from build123d import *

# Parameters (mm, degrees)
F0_R           = 13.97
F0_R_2         = 3.9751
F1_DEPTH       = 15.367
F3_D           = 2.9464
F3_CBORE_D     = 4.572
F3_CBORE_DEPTH = 6.35
F4_R           = 6.4135
F4_R_2         = 3.9751
F5_DEPTH       = 2.54
F6_R           = 1.27
F8_R           = 13.97
F8_R_2         = 12.7
F9_DEPTH       = 10.541


with BuildPart() as f1:
    # F0 (on Front) → F1 (new body)
    with BuildSketch(Plane.XZ):
        Circle(F0_R)
        Circle(F0_R_2, mode=Mode.SUBTRACT)
    extrude(amount=F1_DEPTH)

    # F3 (through all)
    with Locations(Plane.XZ.offset(15.367)):
        with Locations((0, 8.89), (-7.6989658396, -4.445), (7.6989658396, -4.445)):
            CounterBoreHole(F3_D / 2, F3_CBORE_D / 2, F3_CBORE_DEPTH)

    # F4 (on face) → F5 (cut)
    with BuildSketch(Plane(origin=(0, 0, 0), x_dir=(-1, 0, 0), z_dir=(0, 1, 0))):
        Circle(F4_R)
        Circle(F4_R_2, mode=Mode.SUBTRACT)
    extrude(amount=-F5_DEPTH, mode=Mode.SUBTRACT)

    # F7: sweep along a path in F7_path
    with BuildLine(Plane(origin=(13.97, -15.367, 0), x_dir=(0, 0, -1), z_dir=(0, 1, 0))) as f7_path:
        CenterArc((0, 13.97), 13.97, 0, 360)
    # F6 (on Right) → F7 (sweep, cut)
    with BuildSketch(Plane.YZ):
        with Locations((-12.954, 13.97)):
            Circle(F6_R)
    sweep(path=f7_path.line, mode=Mode.SUBTRACT)

    # F8 (on face) → F9 (cut)
    with BuildSketch(Plane(origin=(0, 0, 0), x_dir=(-1, 0, 0), z_dir=(0, 1, 0))):
        Circle(F8_R)
        Circle(F8_R_2, mode=Mode.SUBTRACT)
    extrude(amount=-F9_DEPTH, mode=Mode.SUBTRACT)


solid = f1.part
Geometry check sheet. Reference: the model listing, model coordinates, mm. A direction names the side the tool comes from. Round coordinates to 2 decimals unless told otherwise and drop trailing zeros. Loops run counter-clockwise (first coordinate to the right, second up) from the corner with the lowest first, then second, coordinate; pieces in that order, holes last. Notation, with made-up numbers: (-16, -15) -> (7, -15) arc R14 ccw to (7, -3) -> close; hole circle Ø9 at (-22.5, 45). An arc over 180 degrees is marked (long way). Answer as a JSON object with one key per item and string values. Group by question number.
Item 1: Cross-section at C-C, the plane y = -11.25. Record the cut outline in (x, z) (3 decimals), plus the area to 3 significant figures.
Item 2: Cross-section at A-A, the plane z = 0. Record the cut outline in (x, y), plus the area to 3 significant figures.
Item 3: Cross-section at B-B, the plane x = 0. Record the cut outline in (y, z).
Item 4: Set-up check for faces 1 (the face through (-8.38, -4.45, -5.75)), 2 (the face through (-3, -2.54, 3)), 3 (the face through (-6, -9.017, -4)): record each of +Z, -Z, +X, -X, +Y, -Y from which the full face is reachable in a straight line by a thin tool's end or side.
Item 5: Cross-section at D-D, the plane y = -9.5. Record the cut outline in (x, z) (3 decimals), plus the area to 3 significant figures.
Item 6: Release check for a two-part mould opening along X. For faces 4 (the face through (13.325, -11.104, 4.196)), 5 (the face through (3, -15.367, -3)), 6 (the face through (-6.5, -12.2, -2.5)) record: pulls with the +X half, pulls with the -X half, needs draft (parallel to the pull), parting line crosses it, or undercut.
Item 7: Thickness scan on line 1 along Z through (x, y) = (0, -2); line 2 along Z through (x, y) = (0, -6.5); line 3 along X through (y, z) = (-2.5, -3.75). Record the ranges inside material, lowest first.
Item 8: Depth check by flat-ended pin: pin 1 Ø3.5 at (x, z) = (-7.7, -4.44) entering from -Y; pin 2 Ø12.5 at (x, z) = (0, 0) entering from +Y; pin 3 Ø5 at (x, y) = (-5.5, -4) entering from +Z. Enter the tip coordinate at first touch or a pass-through.
Determined:
{
 "1": {"outline": "circle Ø27.94 at (0, 0); hole circle Ø4.572 at (-7.699, -4.445); hole circle Ø7.95 at (0, 0); hole circle Ø4.572 at (0, 8.89); hole circle Ø4.572 at (7.699, -4.445)", "area": "514 mm²"},
 "2": {"outline": "(-13.97, -15.37) -> (-3.98, -15.37) -> (-3.98, -2.54) -> (-6.41, -2.54) -> (-6.41, 0) -> (-12.7, 0) -> (-12.7, -10.54) -> (-13.97, -10.54) -> (-13.97, -11.68) arc R1.27 cw to (-13.97, -14.22) -> close; (3.98, -15.37) -> (13.97, -15.37) -> (13.97, -14.22) arc R1.27 cw to (13.97, -11.68) -> (13.97, -10.54) -> (12.7, -10.54) -> (12.7, 0) -> (6.41, 0) -> (6.41, -2.54) -> (3.98, -2.54) -> close", "area": "263 mm²"},
 "3": {"outline": "(-15.37, -13.97) -> (-14.22, -13.97) arc R1.27 cw to (-11.68, -13.97) -> (-10.54, -13.97) -> (-10.54, -12.7) -> (0, -12.7) -> (0, -6.41) -> (-2.54, -6.41) -> (-2.54, -3.98) -> (-15.37, -3.98) -> close; (-15.37, 3.98) -> (-2.54, 3.98) -> (-2.54, 6.41) -> (0, 6.41) -> (0, 7.42) -> (-9.02, 7.42) -> (-9.02, 6.6) -> (-15.37, 6.6) -> close; (-15.37, 11.18) -> (-9.02, 11.18) -> (-9.02, 10.36) -> (0, 10.36) -> (0, 12.7) -> (-10.54, 12.7) -> (-10.54, 13.97) -> (-11.68, 13.97) arc R1.27 cw to (-14.22, 13.97) -> (-15.37, 13.97) -> close"},
 "4": {"face 1": "+Y, -Y", "face 2": "+Y", "face 3": "-Y"},
 "5": {"outline": "circle Ø25.4 at (0, 0); hole circle Ø4.572 at (-7.699, -4.445); hole circle Ø7.95 at (0, 0); hole circle Ø4.572 at (0, 8.89); hole circle Ø4.572 at (7.699, -4.445)", "area": "408 mm²"},
 "6": {"face 4": "parting line crosses it", "face 5": "needs draft", "face 6": "undercut"},
 "7": {"line 1": "z = -12.7 to -6.41, 6.41 to 7.42, 10.36 to 12.7", "line 2": "z = -12.7 to -3.98, 3.98 to 7.42, 10.36 to 12.7", "line 3": "x = -12.13 to -9, -6.4 to -5.2, 5.2 to 6.4, 9 to 12.13"},
 "8": {"pin 1": "stops at y = -9.02", "pin 2": "stops at y = -2.54", "pin 3": "stops at z = 12.34"}
}
